For this review, take the finished solid that the model builds, in its own axes (mm). Coordinates: 2 decimals unless noted, no trailing zeros. Loops run counter-clockwise (first coordinate to the right, second up) from the corner with the lowest first, then second, coordinate; pieces in that order, holes last. Notation, with made-up numbers: (74.5, -16) -> (84.5, -16) arc R32 ccw to (84.5, 13) -> close; hole circle Ø2 at (64.5, 39). An arc over 180 degrees is marked (long way). One line per item, written item: value.
from build123d import *

# Parameters (mm, degrees)
BOSS_EXTRUDE1_DEPTH     = 150
SKETCH2_W               = 400
SKETCH2_H               = 65
CUT_EXTRUDE1_DEPTH      = 1
CUT_EXTRUDE1_DEPTH_BACK = 1501
SKETCH3_W               = 600
SKETCH3_H               = 65
CUT_EXTRUDE2_DEPTH      = 130
SKETCH4_R               = 5
BOSS_EXTRUDE2_DEPTH     = 150
SKETCH5_W               = 90
SKETCH5_H               = 75
CUT_EXTRUDE3_DEPTH      = 200
SKETCH6_R               = 15
CUT_EXTRUDE4_DEPTH      = 5
SKETCH7_W               = 180
SKETCH7_H               = 135
CUT_EXTRUDE5_DEPTH      = 120
CUT_EXTRUDE6_START      = -20
SKETCH8_W               = 410
SKETCH8_H               = 110
SKETCH8_R               = 15
CUT_EXTRUDE6_DEPTH      = 200
SKETCH9_W               = 410
SKETCH9_H               = 200
CUT_EXTRUDE7_DEPTH      = 127


with BuildPart() as part:
    # Sketch1 → Boss-Extrude1 (new body)
    with BuildSketch(Plane(origin=(0, 0, 0), x_dir=(1, 0, 0), z_dir=(0, 1, 0))):
        with BuildLine():
            Line((-225, 1000), (-225, 1150))
            Line((-225, 1150), (225, 1150))
            Line((225, 1150), (225, 1000))
            Line((225, 1000), (550, 1000))
            ThreePointArc((550, 1000), (691.421356237, 941.421356237), (750, 800))
            Line((750, 800), (750, -800))
            ThreePointArc((750, -800), (691.421356237, -941.421356237), (550, -1000))
            Line((550, -1000), (-550, -1000))
            ThreePointArc((-550, -1000), (-691.421356237, -941.421356237), (-750, -800))
            Line((-750, -800), (-750, 800))
            ThreePointArc((-750, 800), (-691.421356237, 941.421356237), (-550, 1000))
            Line((-550, 1000), (-225, 1000))
        make_face()
    extrude(amount=BOSS_EXTRUDE1_DEPTH)

    # Sketch2 → Cut-Extrude1 (cut, two sides)
    with BuildSketch(Plane(origin=(750, 0, 0), x_dir=(0, 0, -1), z_dir=(1, 0, 0))) as cut_extrude1_sk:
        with Locations((0, 42.5)):
            Rectangle(SKETCH2_W, SKETCH2_H)
    extrude(amount=CUT_EXTRUDE1_DEPTH, mode=Mode.SUBTRACT)
    extrude(cut_extrude1_sk.sketch, amount=-CUT_EXTRUDE1_DEPTH_BACK, mode=Mode.SUBTRACT)

    # Sketch3 → Cut-Extrude2 (cut)
    with BuildSketch(Plane(origin=(750, 0, 0), x_dir=(0, 0, -1), z_dir=(1, 0, 0))):
        with Locations((500, 42.5)):
            Rectangle(SKETCH3_W, SKETCH3_H)
        with Locations((-500, 42.5)):
            Rectangle(SKETCH3_W, SKETCH3_H)
    cut_extrude2 = extrude(amount=-CUT_EXTRUDE2_DEPTH, mode=Mode.SUBTRACT)

    # Mirror1: Cut-Extrude2 across plane
    add(cut_extrude2.mirror(Plane(origin=(0, 0, 0), x_dir=(0, 0, 1), z_dir=(1, 0, 0))), mode=Mode.SUBTRACT)

    # Sketch4 → Boss-Extrude2 (add)
    with BuildSketch(Plane(origin=(0, 150, 0), x_dir=(1, 0, 0), z_dir=(0, 1, 0))):
        with Locations((-670, 100)):
            Circle(SKETCH4_R)
        with Locations((-670, -100)):
            Circle(SKETCH4_R)
    boss_extrude2 = extrude(amount=-BOSS_EXTRUDE2_DEPTH)

    # Mirror2: Boss-Extrude2 across plane
    add(boss_extrude2.mirror(Plane(origin=(0, 0, 0), x_dir=(0, 0, 1), z_dir=(1, 0, 0))))

    # Sketch5 → Cut-Extrude3 (cut)
    with BuildSketch(Plane.XY.offset(1000)):
        with Locations((-350, 72.5)):
            Rectangle(SKETCH5_W, SKETCH5_H)
        with Locations((350, 72.5)):
            Rectangle(SKETCH5_W, SKETCH5_H)
    extrude(amount=-CUT_EXTRUDE3_DEPTH, mode=Mode.SUBTRACT)

    # Sketch6 → Cut-Extrude4 (cut)
    with BuildSketch(Plane(origin=(0, 0, -1150), x_dir=(-1, 0, 0), z_dir=(0, 0, -1))):
        with Locations((0, 75)):
            Circle(SKETCH6_R)
    extrude(amount=-CUT_EXTRUDE4_DEPTH, mode=Mode.SUBTRACT)

    # Sketch7 → Cut-Extrude5 (cut)
    with BuildSketch(Plane.XY.offset(1000)):
        with Locations((-350, 72.5)):
            Rectangle(SKETCH7_W, SKETCH7_H)
        with Locations((350, 72.5)):
            Rectangle(SKETCH7_W, SKETCH7_H)
    extrude(amount=-CUT_EXTRUDE5_DEPTH, mode=Mode.SUBTRACT)

    # Sketch8 → Cut-Extrude6 (cut)
    with BuildSketch(Plane(origin=(0, 0, -1150), x_dir=(-1, 0, 0), z_dir=(0, 0, -1)).offset(CUT_EXTRUDE6_START)):
        with Locations((0, 75)):
            Rectangle(SKETCH8_W, SKETCH8_H)
        with Locations((0, 75)):
            Circle(SKETCH8_R, mode=Mode.SUBTRACT)
    extrude(amount=-CUT_EXTRUDE6_DEPTH, mode=Mode.SUBTRACT)

    # Sketch9 → Cut-Extrude7 (cut)
    with BuildSketch(Plane(origin=(0, 150, 0), x_dir=(1, 0, 0), z_dir=(0, 1, 0))):
        with Locations((0, 1030)):
            Rectangle(SKETCH9_W, SKETCH9_H)
    extrude(amount=-CUT_EXTRUDE7_DEPTH, mode=Mode.SUBTRACT)


solid = part.part
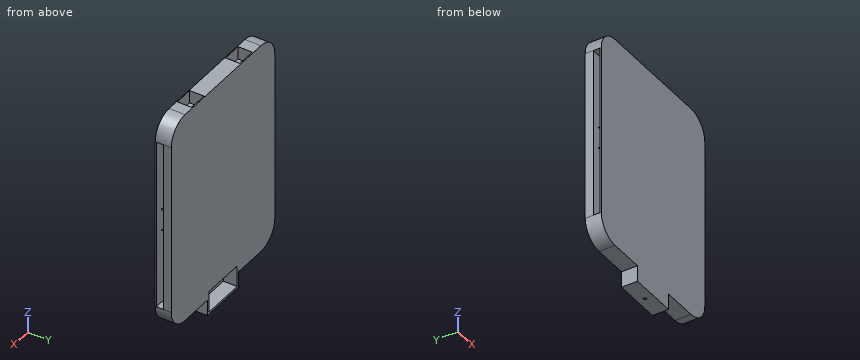
1. Take a section at C-C, the plane z = 697. Give the boundary of the cut face in (x, y), and give its area (3 significant figures).
Return value:
outline: (-750, 0) -> (750, 0) -> (750, 10) -> (620, 10) -> (620, 75) -> (750, 75) -> (750, 150) -> (-750, 150) -> (-750, 75) -> (-620, 75) -> (-620, 10) -> (-750, 10) -> close
area: 208,000 mm2
2. Take a section at D-D, the plane x = 357.5. Give the boundary of the cut face in (y, z), and give its area (3 significant figures).
Return value:
outline: (0, -1000) -> (150, -1000) -> (150, 1000) -> (140, 1000) -> (140, 880) -> (110, 880) -> (110, 800) -> (35, 800) -> (35, 880) -> (5, 880) -> (5, 1000) -> (0, 1000) -> close; hole (10, -200) -> (75, -200) -> (75, 200) -> (10, 200) -> close
area: 252,000 mm2
3. To check wall thickness, follow probe 1 along Z at (x, y) = (134, 64); probe 2 along Y at (x, z) = (-639.5, -774); probe 3 along Z at (x, y) = (62, 81). State the ranges of each line that lie inside material, in increasing order. Write a range as from..to.
Return value:
probe 1: z = -1150..-1130, -930..-200, 200..1000
probe 2: y = 0..10, 75..150
probe 3: z = -1150..-1130, -930..1000
4. Take a section at B-B, the plane z = 144.5. Give the boundary of the cut face in (x, y).
Return value:
outline: (-750, 0) -> (750, 0) -> (750, 10) -> (-750, 10) -> close; (-750, 75) -> (750, 75) -> (750, 150) -> (-750, 150) -> close
5. Take a section at A-A, the plane x = 71.5. Give the boundary of the cut face in (y, z), and give its area (4 significant figures).
Return value:
outline: (0, -1150) -> (150, -1150) -> (150, -1130) -> (20, -1130) -> (20, -930) -> (150, -930) -> (150, 1000) -> (0, 1000) -> close; hole (10, -200) -> (75, -200) -> (75, 200) -> (10, 200) -> close
area: 270,500 mm2
6. Insertion check: pin 1 Ø2 at (x, y) = (598.5, 59.5) entering from -Z; pin 2 Ø19.5 at (x, y) = (-699.5, 28.5) entering from +Z; pin 3 Ø1 at (y, z) = (94, -816.5) entering from -X. Each pin has a flat end and moves straight along its axis. Give the tip position at first contact, or say it passes through.
Return value:
pin 1: stops at z = -994.28
pin 2: stops at z = 943.07
pin 3: stops at x = -749.36
